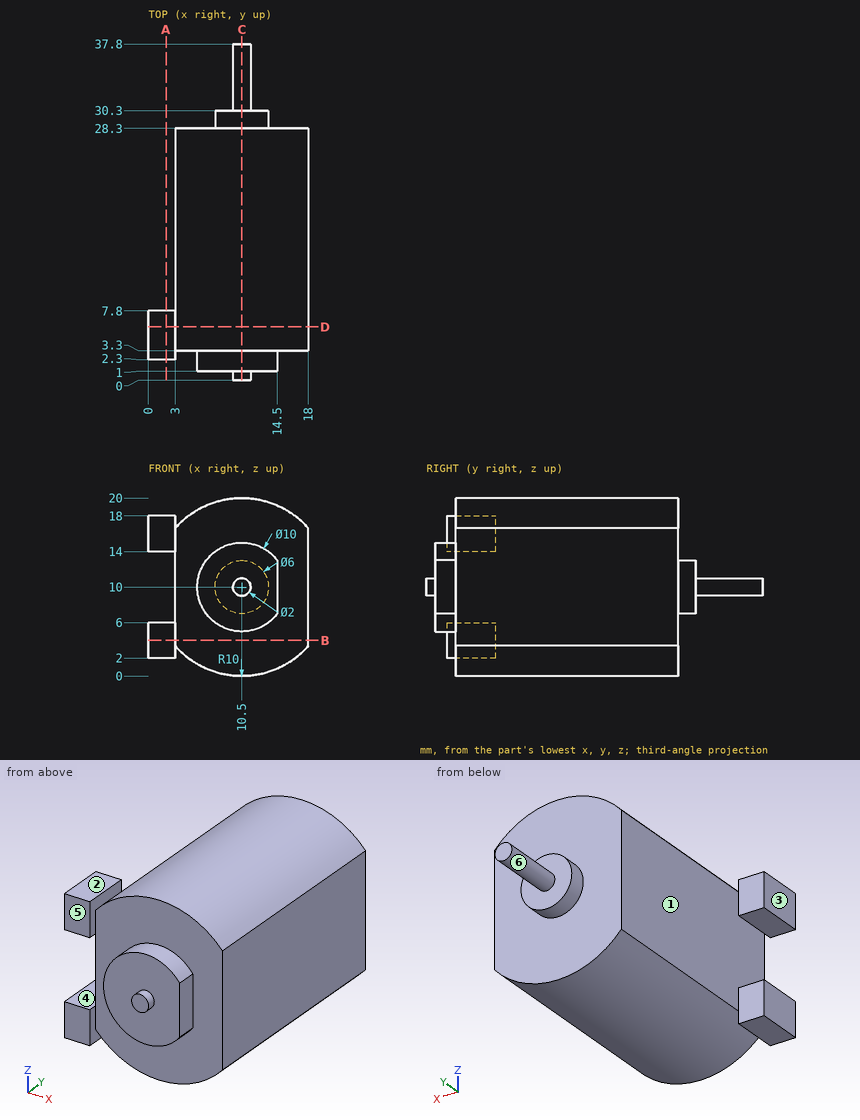
The drawing under review shows one solid part. Ordinate dimensions are in mm from its lowest x, y, z. A direction names the side the tool comes from. Round coordinates to 2 decimals unless told otherwise and drop trailing zeros. Write each loop counter-clockwise with the first axis right and the second up, starting at its lowest first coordinate (ties: lowest second). Pieces come first, ordered by that corner, then holes. Notation, with made-up numbers: (2, 61) - (41, 61) arc R12 cw to (41, 79) - close; hole circle Ø4 at (31.5, 11). An arc over 180 degrees is marked (long way). Put each result on its own line as item: value.
Q1. We need section D-D (y = 6). Give the boundary of the cut face in (x, z), and give its area (3 significant figures).
Solved:
outline: (0, 2) - (3, 2) - (3, 3.39) arc R10 ccw to (18, 3.39) - (18, 16.61) arc R10 ccw to (3, 16.61) - (3, 18) - (0, 18) - (0, 14) - (3, 14) - (3, 6) - (0, 6) - close
area: 293 mm2
Q2. We need section B-B (z = 4). Give the boundary of the cut face in (x, y), and give its area (4 significant figures).
Solved:
outline: (0, 2.3) - (3, 2.3) - (3, 3.3) - (18, 3.3) - (18, 28.3) - (3, 28.3) - (3, 7.8) - (0, 7.8) - close
area: 391.5 mm2
Q3. We need section C-C (x = 10.5). Give the boundary of the cut face in (y, z), and give its area (3 significant figures).
Solved:
outline: (0, 9) - (1, 9) - (1, 5) - (3.3, 5) - (3.3, 0) - (28.3, 0) - (28.3, 7) - (30.3, 7) - (30.3, 9) - (37.8, 9) - (37.8, 11) - (30.3, 11) - (30.3, 13) - (28.3, 13) - (28.3, 20) - (3.3, 20) - (3.3, 15) - (1, 15) - (1, 11) - (0, 11) - close
area: 552 mm2
Q4. Insertion check: pin 1 Ø5 at (x, y) = (4.5, 21) entering from +Z; pin 2 Ø7.5 at (x, z) = (7, 11) entering from +Y; pin 3 Ø1.5 at (x, y) = (2, 5) entering from +Z; pin 4 Ø3.5 at (x, y) = (1, 5) entering from -Z. Each pin has a flat end and moves straight along its axis. Give the tip position at first contact, or say it passes through.
Solved:
pin 1: stops at z = 19.37
pin 2: stops at y = 37.8
pin 3: stops at z = 18
pin 4: stops at z = 2
Q5. Machinability: for the marked faces 4, 5 and 6, which of the approach directions +Z, -Z, +X, -X, +Y, -Y give a long, thin tool a straight path to every point of the face, cutting with its end or side? Answer none if there is none.
Solved:
face 4: -X, +Y, -Y
face 5: +Z, -Z, -X, -Y
face 6: +Y
Q6. Wall thickness on probe 1 along Y at (x, z) = (4.75, 4.25); probe 2 along X at (y, z) = (18, 6.75); probe 3 along Y at (x, z) = (10, 6.25): over which ranges is each line inside the solid? List them lowest first.
Solved:
probe 1: y = 3.3 to 28.3
probe 2: x = 3 to 18
probe 3: y = 1 to 28.3
Q7. Mouldability with a two-part tool opening along Z and no side actions: class the marked faces 1, 2 and 3 as released by +Z, released by -Z, zero draft, split by the parting line, or undercut.
Solved:
face 1: undercut
face 2: released by +Z
face 3: zero draft
Q8. We need section A-A (x = 2). Give the boundary of the cut face in (y, z), and give its area (3 significant figures).
Solved:
outline: (2.3, 2) - (7.8, 2) - (7.8, 6) - (2.3, 6) - close; (2.3, 14) - (7.8, 14) - (7.8, 18) - (2.3, 18) - close
area: 44.0 mm2
